```python
from build123d import *

# Parameters (mm, degrees)
SKETCH1_W           = 140
SKETCH1_H           = 70
BOSS_EXTRUDE1_DEPTH = 5
SKETCH2_R           = 2.25
CUT_EXTRUDE1_DEPTH  = 145.395290782
SKETCH3_W           = 51
SKETCH3_H           = 51
CUT_EXTRUDE2_DEPTH  = 0.5
SKETCH4_W           = 47
SKETCH4_H           = 47
CUT_EXTRUDE3_DEPTH  = 79.89866919
SKETCH5_W           = 10
SKETCH5_H           = 5
SKETCH5_W_2         = 5
SKETCH5_H_2         = 10
CUT_EXTRUDE4_DEPTH  = 79.89866919


with BuildPart() as part:
    # Sketch1 → Boss-Extrude1 (new, symmetric)
    with BuildSketch(Plane(origin=(0, 0, 0), x_dir=(1, 0, 0), z_dir=(0, 1, 0))):
        Rectangle(SKETCH1_W, SKETCH1_H)
    extrude(amount=BOSS_EXTRUDE1_DEPTH, both=True)

    # Sketch2 → Cut-Extrude1 (cut, through all)
    with BuildSketch(Plane(origin=(70, 0, 0), x_dir=(0, 0, -1), z_dir=(1, 0, 0))):
        with Locations((-30, 0)):
            Circle(SKETCH2_R)
        with Locations((30, 0)):
            Circle(SKETCH2_R)
    extrude(amount=-CUT_EXTRUDE1_DEPTH, mode=Mode.SUBTRACT)

    # Sketch3 → Cut-Extrude2 (cut, symmetric)
    with BuildSketch(Plane(origin=(0, 0, 0), x_dir=(1, 0, 0), z_dir=(0, 1, 0))):
        with Locations((-35, 0)):
            Rectangle(SKETCH3_W, SKETCH3_H)
    cut_extrude2 = extrude(amount=CUT_EXTRUDE2_DEPTH, both=True, mode=Mode.SUBTRACT)

    # Sketch4 → Cut-Extrude3 (cut, through all)
    with BuildSketch(Plane(origin=(0, 5, 0), x_dir=(1, 0, 0), z_dir=(0, 1, 0))):
        with Locations((-35, 0)):
            Rectangle(SKETCH4_W, SKETCH4_H)
    cut_extrude3 = extrude(amount=-CUT_EXTRUDE3_DEPTH, mode=Mode.SUBTRACT)

    # Sketch5 → Cut-Extrude4 (cut, through all)
    with BuildSketch(Plane(origin=(0, 5, 0), x_dir=(1, 0, 0), z_dir=(0, 1, 0))):
        with Locations((-47.5, 26)):
            Rectangle(SKETCH5_W, SKETCH5_H)
        with Locations((-22.5, 26)):
            Rectangle(SKETCH5_W, SKETCH5_H)
        with Locations((-9, 12.5)):
            Rectangle(SKETCH5_W_2, SKETCH5_H_2)
        with Locations((-9, -12.5)):
            Rectangle(SKETCH5_W_2, SKETCH5_H_2)
        with Locations((-22.5, -26)):
            Rectangle(SKETCH5_W, SKETCH5_H)
        with Locations((-47.5, -26)):
            Rectangle(SKETCH5_W, SKETCH5_H)
        with Locations((-61, -12.5)):
            Rectangle(SKETCH5_W_2, SKETCH5_H_2)
        with Locations((-61, 12.5)):
            Rectangle(SKETCH5_W_2, SKETCH5_H_2)
    cut_extrude4 = extrude(amount=-CUT_EXTRUDE4_DEPTH, mode=Mode.SUBTRACT)

    # Mirror1: Cut-Extrude2, Cut-Extrude3, Cut-Extrude4 across plane
    add(cut_extrude2.mirror(Plane(origin=(0, 0, 0), x_dir=(0, 0, 1), z_dir=(1, 0, 0))), mode=Mode.SUBTRACT)
    add(cut_extrude3.mirror(Plane(origin=(0, 0, 0), x_dir=(0, 0, 1), z_dir=(1, 0, 0))), mode=Mode.SUBTRACT)
    add(cut_extrude4.mirror(Plane(origin=(0, 0, 0), x_dir=(0, 0, 1), z_dir=(1, 0, 0))), mode=Mode.SUBTRACT)


solid = part.part
```
Model file for the job. Use its own axes, mm. A direction names the side the tool comes from. Round coordinates to 2 decimals unless told otherwise and drop trailing zeros. Order: outer loops, then holes, each group sorted by start corner. A loop starts at its lowest first (then second) coordinate and runs counter-clockwise, first axis right, second up. Notation, with made-up numbers: M 45.25,42 L 66.25,42 A30 ccw 66.25,80 Z; hole C 87.5,22.5 d1. An arc over 180 degrees is marked long. Use CSV: the item, a comma, the result in double quotes.
Item 1: Saw through at A-A (x = 40.5). List the corners of the cut face in (y, z).
Worked answers:
outline,"M -5,-35 L 5,-35 L 5,-23.5 L 0.5,-23.5 L 0.5,-25.5 L -0.5,-25.5 L -0.5,-23.5 L -5,-23.5 Z; M -5,23.5 L -0.5,23.5 L -0.5,25.5 L 0.5,25.5 L 0.5,23.5 L 5,23.5 L 5,35 L -5,35 Z; hole C 0,-30 d4.5; hole C 0,30 d4.5"
Item 2: Which spindle directions (+Z, -Z, +X, -X, +Y, -Y) get a long thin tool onto all of the face, cutting with end or side? Do faces 4 (the face through (-15, -3, 23.5)), 5 (the face through (-1, 0, -35)), 6 (the face through (-59, 0.5, 23)). Say none if no direction does.
Worked answers:
face 4,"+Y, -Y"
face 5,"-Z, +X, -X, +Y, -Y"
face 6,"none"
Item 3: Pull direction Y, two halves, no side cores. Call faces 1 (the face through (-1, 5, 0)), 2 (the face through (-23, -3, 28.5)), 3 (the face through (59, 0.5, -23)): released by +Y, released by -Y, zero draft, split by the parting line, or undercut.
Worked answers:
face 1,"released by +Y"
face 2,"zero draft"
face 3,"undercut"
Item 4: Saw through at D-D (x = -47). List the corners of the cut face in (y, z).
Worked answers:
outline,"M -5,-35 L 5,-35 L 5,-28.5 L 1.68,-28.5 A2.25 cw long -1.68,-28.5 L -5,-28.5 Z; M -5,28.5 L -1.68,28.5 A2.25 cw long 1.68,28.5 L 5,28.5 L 5,35 L -5,35 Z"
Item 5: Saw through at C-C (z = 13.5). List the corners of the cut face in (x, y).
Worked answers:
outline,"M -70,-5 L -63.5,-5 L -63.5,5 L -70,5 Z; M -6.5,-5 L 6.5,-5 L 6.5,5 L -6.5,5 Z; M 63.5,-5 L 70,-5 L 70,5 L 63.5,5 Z"
Item 6: Probe probe 1 along X at (y, z) = (0.25, -8.5); probe 2 along X at (y, z) = (-2.25, 24); probe 3 along X at (y, z) = (-2.75, 7). List the from-to ranges inside material, lowest first.
Worked answers:
probe 1,"-70 to -63.5, -6.5 to 6.5, 63.5 to 70"
probe 2,"-70 to -52.5, -42.5 to -27.5, -17.5 to 17.5, 27.5 to 42.5, 52.5 to 70"
probe 3,"-70 to -58.5, -11.5 to 11.5, 58.5 to 70"
Item 7: Saw through at B-B (z = 30). List the corners of the cut face in (x, y).
Worked answers:
outline,"M -70,-5 L 70,-5 L 70,-2.25 L -70,-2.25 Z; M -70,2.25 L 70,2.25 L 70,5 L -70,5 Z"
